Can you work these out from the model? Positions are in its coordinate system, mm. Give positions to 0.01 mm unless a question says otherwise; leave off trailing zeros. Loops run counter-clockwise (first coordinate to the right, second up) from the corner with the lowest first, then second, coordinate; pieces in that order, holes last.
from build123d import *

# Parameters (mm, degrees)
BOSS_EXTRUDE1_DEPTH     = 1.984375
F_1_4_28_TAPPED_HOLE1_D = 5.4102
SKETCH5_OUTSIDE_W       = 33.81
SKETCH5_OUTSIDE_H       = 35.53
SKETCH5_OUTSIDE_R       = 5.55625
CUT_EXTRUDE2_DEPTH      = 4.96875
CUT_EXTRUDE2_TAPER      = 60


with BuildPart() as part:
    # Sketch1 → Boss-Extrude1 (new body, symmetric)
    with BuildSketch(Plane(origin=(0, 0, 0), x_dir=(1, 0, 0), z_dir=(0, 1, 0))):
        Polygon((-5.55625, 3.207902433), (-5.55625, -3.207902433), (0, -6.415804866), (5.55625, -3.207902433), (5.55625, 3.207902433), (0, 6.415804866), align=None)
    extrude(amount=BOSS_EXTRUDE1_DEPTH, both=True)

    # 1/4-28 Tapped Hole1 (through all)
    with Locations(Plane(origin=(0, 1.984375, 0), x_dir=(1, 0, 0), z_dir=(0, 1, 0))):
        with Locations((0, 0)):
            Hole(F_1_4_28_TAPPED_HOLE1_D / 2)

    # Sketch5 outside → Cut-Extrude2 (cut, through all)
    with BuildSketch(Plane(origin=(0, 1.984375, 0), x_dir=(1, 0, 0), z_dir=(0, 1, 0))):
        Rectangle(SKETCH5_OUTSIDE_W, SKETCH5_OUTSIDE_H)
        Circle(SKETCH5_OUTSIDE_R, mode=Mode.SUBTRACT)
    cut_extrude2 = extrude(amount=-CUT_EXTRUDE2_DEPTH, taper=CUT_EXTRUDE2_TAPER, mode=Mode.SUBTRACT)

    # Mirror1: Cut-Extrude2 across plane
    add(cut_extrude2.mirror(Plane.ZX), mode=Mode.SUBTRACT)


solid = part.part
(1) Please list where these lines run through material, in increasing order: probe 1 along X at (y, z) = (-0.8, -0.25); probe 2 along Z at (x, y) = (-1, -0.45); probe 3 along X at (y, z) = (-0.05, -1).
Returned:
probe 1: x = -5.56 to -2.69, 2.69 to 5.56
probe 2: z = -5.84 to -2.51, 2.51 to 5.84
probe 3: x = -5.56 to -2.51, 2.51 to 5.56
(2) Will these pins go through, and if not, where does the flat tip stop? P1, Ø1.5, axis at y = -1, z = 4.5, coming from the +X side; P2, Ø1.5, axis at x = -3, y = -1, coming from the -Z side.
Returned:
P1: stops at x = 4.62
P2: stops at z = -5.12
(3) Suppose I cut it at A-A on y = 0. List the corners of the cut face in (x, z) for me.
Returned:
outline: (-5.56, -3.21) - (0, -6.42) - (5.56, -3.21) - (5.56, 3.21) - (0, 6.42) - (-5.56, 3.21) - close; hole circle Ø5.41 at (0, 0)
